Can you work these out from the model? Positions are in its coordinate system, mm. Face numbers are marked on the shaded views. A direction names the side the tool comes from. Round coordinates to 2 decimals unless told otherwise and drop trailing zeros. Order: outer loops, then holes, each group sorted by start corner. A loop starts at its lowest first (then second) coordinate and runs counter-clockwise, first axis right, second up.
Q1. If we section it at C-C (z = -1.5): Please give me the cut outline in (x, y), plus the area to 3 significant figures.
Q2. Will these pins go through, and if not, where does the flat tip stop? P1, Ø6, axis at y = -3.5, z = -0.5, coming from the -X side; P2, Ø3.5, axis at x = 0, z = 2, coming from the -Y side.
Q3. If we section it at A-A (x = 0): Count the separate pieces of the cut face and the enclosed holes in it, plus the area to 3 significant figures.
Q4. For the marked faces 1 and 2, which set-ups out of +Z, -Z, +X, -X, +Y, -Y let a thin tool reach every point of the face, with its end or its side?
Q5. If I drill on line 1 (Y direction, x = 0, z = 10.4); line 2 (X direction, y = 1.15, z = 0) (3 decimals); line 3 (Y direction, x = -1.5, z = 10.25), over which ranges is the centre line in solid material (lowest first)?
Q6. If we section it at B-B (y = -37): Please give me the cut outline in (x, z).
Q7. We'd pull the mould along X, two halves only. Please class the marked faces 3, 4, 5 and 6: pulls with the +X half, pulls with the -X half, needs draft (parallel to the pull), parting line crosses it, or undercut.
Q8. If we section it at D-D (y = -28.5): Please give me the cut outline in (x, z), plus the area to 3 significant figures.
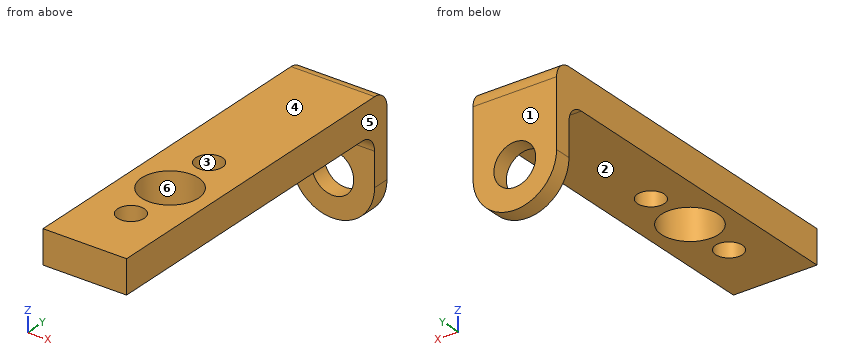
from build123d import *

# Parameters (mm, degrees)
SKETCH2_R           = 3.175
BOSS_EXTRUDE1_DEPTH = 2.54
SKETCH4_W           = 12.7
SKETCH4_H           = 5.08
BOSS_EXTRUDE2_DEPTH = 50.8
FILLET1_R           = 2.54
FILLET2_R           = 2.54
SKETCH5_R           = 4.318
SKETCH5_R_2         = 2.032
CUT_EXTRUDE1_DEPTH  = 55.624765446
CIRPATTERN1_COUNT   = 2


with BuildPart() as part:
    # Sketch2 → Boss-Extrude1 (new body)
    with BuildSketch(Plane(origin=(0, 0, 0), x_dir=(1, 0, 0), z_dir=(0, 1, 0))):
        with BuildLine():
            Line((-6.35, 0), (-6.35, -12.7))
            Line((-6.35, -12.7), (6.35, -12.7))
            Line((6.35, -12.7), (6.35, 0))
            ThreePointArc((6.35, 0), (0, 6.35), (-6.35, 0))
        make_face()
        with Locations(Location((0, 0, 0), (0, 0, 270))):
            Circle(SKETCH2_R, mode=Mode.SUBTRACT)
    extrude(amount=BOSS_EXTRUDE1_DEPTH)

    # Sketch4 → Boss-Extrude2 (add)
    with BuildSketch(Plane.XZ):
        with Locations((0, 10.16)):
            Rectangle(SKETCH4_W, SKETCH4_H)
    extrude(amount=BOSS_EXTRUDE2_DEPTH)

    # Fillet1
    fillet1_edges = [part.edges().sort_by_distance(p)[0] for p in [
        (0, 2.54, 12.7),
    ]]
    fillet(fillet1_edges, radius=FILLET1_R)

    # Fillet2
    fillet2_edges = [part.edges().sort_by_distance(p)[0] for p in [
        (0, 0, 7.62),
    ]]
    fillet(fillet2_edges, radius=FILLET2_R)

    # Sketch5 → Cut-Extrude1 (cut, through all)
    with BuildSketch(Plane.XY.offset(12.7)):
        with Locations((0, -33.3375)):
            Circle(SKETCH5_R)
        with Locations((0, -25.3365)):
            Circle(SKETCH5_R_2)
    cut_extrude1 = extrude(amount=-CUT_EXTRUDE1_DEPTH, mode=Mode.SUBTRACT)

    # CirPattern1: Cut-Extrude1 ×2 about axis
    cirpattern1_axis = Axis((0, -33.3375, 0), (0, 0, 1))
    for i in range(1, CIRPATTERN1_COUNT):
        add(cut_extrude1.rotate(cirpattern1_axis, i * 360 / CIRPATTERN1_COUNT), mode=Mode.SUBTRACT)


solid = part.part
Solution:
1. outline: (-6.17, 0) - (-2.8, 0) - (-2.8, 2.54) - (-6.17, 2.54) - close; (2.8, 0) - (6.17, 0) - (6.17, 2.54) - (2.8, 2.54) - close
1. area: 17.1 mm2
2. P1: passes through
2. P2: stops at y = 0
3. separate pieces: 5
3. enclosed holes: 0
3. area: 205 mm2
4. face 1: +Z, -Z, +X, -X, +Y
4. face 2: -Z, +X, -X, -Y
5. line 1: y = -50.8 to -43.37, -39.31 to -37.66, -29.02 to -27.37, -23.3 to 2.53
5. line 2: x = -6.35 to -3.175, 3.175 to 6.35
5. line 3: y = -50.8 to -42.71, -39.97 to -37.39, -29.29 to -26.71, -23.97 to 2.54
6. outline: (-6.35, 7.62) - (-2.29, 7.62) - (-2.29, 12.7) - (-6.35, 12.7) - close; (2.29, 7.62) - (6.35, 7.62) - (6.35, 12.7) - (2.29, 12.7) - close
7. face 3: undercut
7. face 4: needs draft
7. face 5: pulls with the +X half
7. face 6: undercut
8. outline: (-6.35, 7.62) - (6.35, 7.62) - (6.35, 12.7) - (-6.35, 12.7) - close
8. area: 64.5 mm2
